Source: CAD feature listing. Evaluate the final solid. Frame: model axes, mm. Face numbers are marked on the shaded views. A direction names the side the tool comes from. Round coordinates to 2 decimals unless told otherwise and drop trailing zeros. Order: outer loops, then holes, each group sorted by start corner. A loop starts at its lowest first (then second) coordinate and runs counter-clockwise, first axis right, second up. Notation, with made-up numbers: (21.5, -18.5) - (29.5, -18.5) arc R19 cw to (29.5, -10.5) - close; hole circle Ø11 at (-22.75, -16). An arc over 180 degrees is marked (long way). Use one line per item in the form item = value. Start each with the question number.
Q1. Ray query, line 1 (Y direction, x = 20, z = 1.05); line 2 (X direction, y = -0.5, z = 1.4). Return the intervals inside material, ascending. Write a range as [from, to].
Q2. Cut plane D-D, the plane x = 1. Return the cut outline in (y, z).
Q3. Cut plane B-B, the plane y = 0. Return the cut outline in (x, z), and give its area (3 significant figures).
Q4. Set-up query: the marked faces 1, 2 and 3. Return all of +Z, -Z, +X, -X, +Y, -Y with unobstructed straight access to the full face (end or side cutting, diameter ignored); none if empty.
Q5. Pin query (flat end, axial travel): pin 1 Ø1 at (y, z) = (3, 0.5) entering from -X; pin 2 Ø1 at (y, z) = (0.5, -1.5) entering from -X; pin 3 Ø3 at (x, y) = (6, 0) entering from -Z. Return the tip coordinate at first contact, or that it passes through.
Q6. Cut plane C-C, the plane z = 0.85. Return the cut outline in (x, y).
Q7. Cut plane A-A, the plane x = 26. Return the cut outline in (y, z), and give its area (3 significant figures).
from build123d import *

# Parameters (mm, degrees)
ESBO_O1_R                = 1.75
RESSALTO_EXTRUS_O1_DEPTH = 2
ESBO_O2_W                = 2
ESBO_O2_H                = 10
RESSALTO_EXTRUS_O2_DEPTH = 2


with BuildPart() as part:
    # Esboço1 → Ressalto-extrusão1 (new body)
    with BuildSketch(Plane.XY):
        with BuildLine():
            Line((0, 5), (35, 5))
            ThreePointArc((35, 5), (40, 0), (35, -5))
            Line((35, -5), (0, -5))
            ThreePointArc((0, -5), (-5, 0), (0, 5))
        make_face()
        Circle(ESBO_O1_R, mode=Mode.SUBTRACT)
        with BuildLine():
            Line((20, 1.75), (35, 1.75))
            ThreePointArc((35, 1.75), (36.75, 0), (35, -1.75))
            Line((35, -1.75), (20, -1.75))
            ThreePointArc((20, -1.75), (18.25, 0), (20, 1.75))
        make_face(mode=Mode.SUBTRACT)
    extrude(amount=RESSALTO_EXTRUS_O1_DEPTH)

    # Esboço2 → Ressalto-extrusão2 (add)
    with BuildSketch(Plane(origin=(0, 0, 0), x_dir=(-1, 0, 0), z_dir=(0, 0, -1))):
        with Locations((-16.2, 0)):
            Rectangle(ESBO_O2_W, ESBO_O2_H)
    extrude(amount=RESSALTO_EXTRUS_O2_DEPTH)


solid = part.part
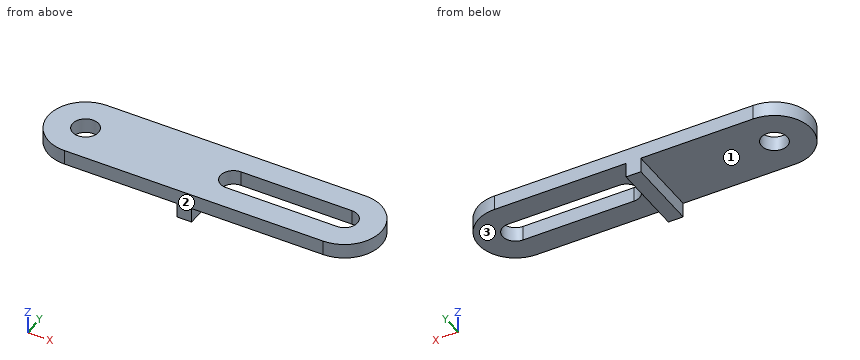
Completed:
q1.line_1 = [-5, -1.75], [1.75, 5]
q1.line_2 = [-4.97, -1.68], [1.68, 18.32], [36.68, 39.97]
q2.outline = (-5, 0) - (-1.44, 0) - (-1.44, 2) - (-5, 2) - close; (1.44, 0) - (5, 0) - (5, 2) - (1.44, 2) - close
q3.outline = (-5, 0) - (-1.75, 0) - (-1.75, 2) - (-5, 2) - close; (1.75, 0) - (15.2, 0) - (15.2, -2) - (17.2, -2) - (17.2, 0) - (18.25, 0) - (18.25, 2) - (1.75, 2) - close; (36.75, 0) - (40, 0) - (40, 2) - (36.75, 2) - close
q3.area = 50.0 mm2
q4.face_1 = -Z, -X, +Y, -Y
q4.face_2 = +Z, -Z, +X, -X, -Y
q4.face_3 = -Z, +X, +Y, -Y
q5.pin_1 = -4.33
q5.pin_2 = 15.2
q5.pin_3 = 0
q6.outline = (0, -5) - (35, -5) arc R5 ccw to (35, 5) - (0, 5) arc R5 ccw to start; hole circle Ø3.5 at (0, 0); hole (20, -1.75) - (35, -1.75) arc R1.75 ccw to (35, 1.75) - (20, 1.75) arc R1.75 ccw to start
q7.outline = (-5, 0) - (-1.75, 0) - (-1.75, 2) - (-5, 2) - close; (1.75, 0) - (5, 0) - (5, 2) - (1.75, 2) - close
q7.area = 13.0 mm2
